Geometry: final body of the model. Coordinates: model frame, mm. Face numbers are marked on the shaded views. Round coordinates to 2 decimals unless told otherwise and drop trailing zeros. Order: outer loops, then holes, each group sorted by start corner. A loop starts at its lowest first (then second) coordinate and runs counter-clockwise, first axis right, second up. Notation, with made-up numbers: M 74,1 L 122,1 A20 ccw 122,12 Z; hole C 59,78.5 d6. An arc over 180 degrees is marked long. Put each result on its own line as item: value. Start each with the question number.
1) Material intervals for probe 1 along Y at (x, z) = (0, -0.75); probe 2 along Y at (x, z) = (-1.5, -0.4); probe 3 along X at (y, z) = (3, -2.3), sorted ascending. Write a range as [from, to].
2) Section D-D, the plane z = -1.9. Count the separate pieces of the cut face and the enclosed holes in it, then the cut area to 3 significant figures.
3) Draft query along Y for the marked faces 1, 2 and 3. Return one class per face: pulls with the +Y half, pulls with the -Y half, needs draft (parallel to the pull), parting line crosses it, or undercut.
4) Section A-A, the plane x = 0. Return loops of the section in (y, z).
5) Section B-B, the plane y = -4.5. Return loops of the section in (x, z), then the cut area to 3 significant figures.
6) Section C-C, the plane x = -11. Return loops of the section in (y, z).
7) First-contact query: P1, Ø1, axis at x = 12.5, z = -1, coming from the -Y side; P2, Ø1.5, axis at y = 1.5, z = -1.5, coming from the +X side. Flat tips, straight axial feed; report the tip coordinate or a pass-through.
from build123d import *

# Parameters (mm, degrees)
F0_R     = 13.5
F0_R_2   = 2
F1_DEPTH = 2.75
F2_R     = 5


with BuildPart() as f1:
    # F0 (on Top) → F1 (new body)
    with BuildSketch(Plane.XY):
        with BuildLine():
            ThreePointArc((-4, 18.0623918682), (-11.5812348219, -14.4265380463), (18.5, 0))
            ThreePointArc((18.5, 0), (14.4265380463, 11.5812348219), (4, 18.0623918682))
            ThreePointArc((4, 18.0623918682), (3.2273401507, 18.2163189353), (2.4488272709, 18.3372093023))
            ThreePointArc((2.4488272709, 18.3372093023), (0, 17.5), (-2.4488272709, 18.3372093023))
            ThreePointArc((-2.4488272709, 18.3372093023), (-3.2273401507, 18.2163189353), (-4, 18.0623918682))
        make_face()
        Circle(F0_R, mode=Mode.SUBTRACT)
        with BuildLine():
            ThreePointArc((-2.4488272709, 18.3372093023), (0, 17.5), (2.4488272709, 18.3372093023))
            ThreePointArc((2.4488272709, 18.3372093023), (0, 18.5), (-2.4488272709, 18.3372093023))
        make_face()
        with BuildLine():
            ThreePointArc((-2.4488272709, 18.3372093023), (0, 18.5), (2.4488272709, 18.3372093023))
            ThreePointArc((2.4488272709, 18.3372093023), (3.5913304696, 19.7386523744), (4, 21.5))
            ThreePointArc((4, 21.5), (0, 25.5), (-4, 21.5))
            ThreePointArc((-4, 21.5), (-3.5913304696, 19.7386523744), (-2.4488272709, 18.3372093023))
        make_face()
        with Locations((0, 21.5)):
            Circle(F0_R_2, mode=Mode.SUBTRACT)
        with BuildLine():
            ThreePointArc((2.4488272709, 18.3372093023), (3.2273401507, 18.2163189353), (4, 18.0623918682))
            Line((4, 18.0623918682), (4, 21.5))
            ThreePointArc((4, 21.5), (3.5913304696, 19.7386523744), (2.4488272709, 18.3372093023))
        make_face()
        with BuildLine():
            Line((-4, 21.5), (-4, 18.0623918682))
            ThreePointArc((-4, 18.0623918682), (-3.2273401507, 18.2163189353), (-2.4488272709, 18.3372093023))
            ThreePointArc((-2.4488272709, 18.3372093023), (-3.5913304696, 19.7386523744), (-4, 21.5))
        make_face()
    extrude(amount=-F1_DEPTH)

    # F2
    f2_edges = [f1.edges().sort_by_distance(p)[0] for p in [
        (4, 18.062392, -1.375),
        (-4, 18.062392, -1.375),
    ]]
    fillet(f2_edges, radius=F2_R)


solid = f1.part
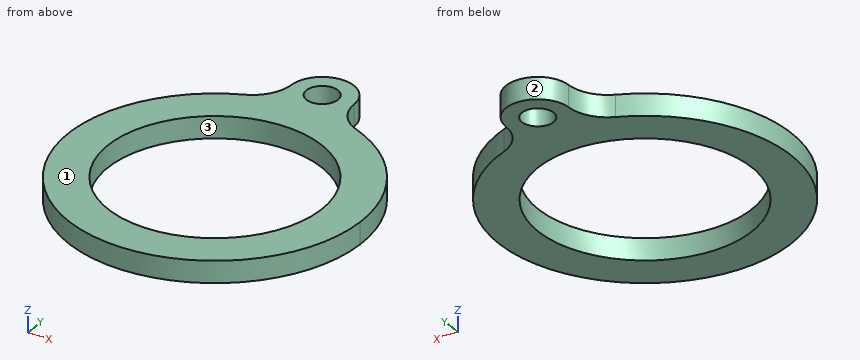
Result sheet:
1. probe 1: y = [-18.5, -13.5], [13.5, 19.5], [23.5, 25.5]
1. probe 2: y = [-18.44, -13.42], [13.42, 20.18], [22.82, 25.21]
1. probe 3: x = [-18.26, -13.16], [13.16, 18.26]
2. separate pieces: 1
2. enclosed holes: 2
2. area: 545 mm2
3. face 1: needs draft
3. face 2: pulls with the +Y half
3. face 3: undercut
4. outline: M -18.5,-2.75 L -13.5,-2.75 L -13.5,0 L -18.5,0 Z; M 13.5,-2.75 L 19.5,-2.75 L 19.5,0 L 13.5,0 Z; M 23.5,-2.75 L 25.5,-2.75 L 25.5,0 L 23.5,0 Z
5. outline: M -17.94,-2.75 L -12.73,-2.75 L -12.73,0 L -17.94,0 Z; M 12.73,-2.75 L 17.94,-2.75 L 17.94,0 L 12.73,0 Z
5. area: 28.7 mm2
6. outline: M -14.87,-2.75 L -7.83,-2.75 L -7.83,0 L -14.87,0 Z; M 7.83,-2.75 L 14.87,-2.75 L 14.87,0 L 7.83,0 Z
7. P1: stops at y = -14.08
7. P2: stops at x = 18.48
